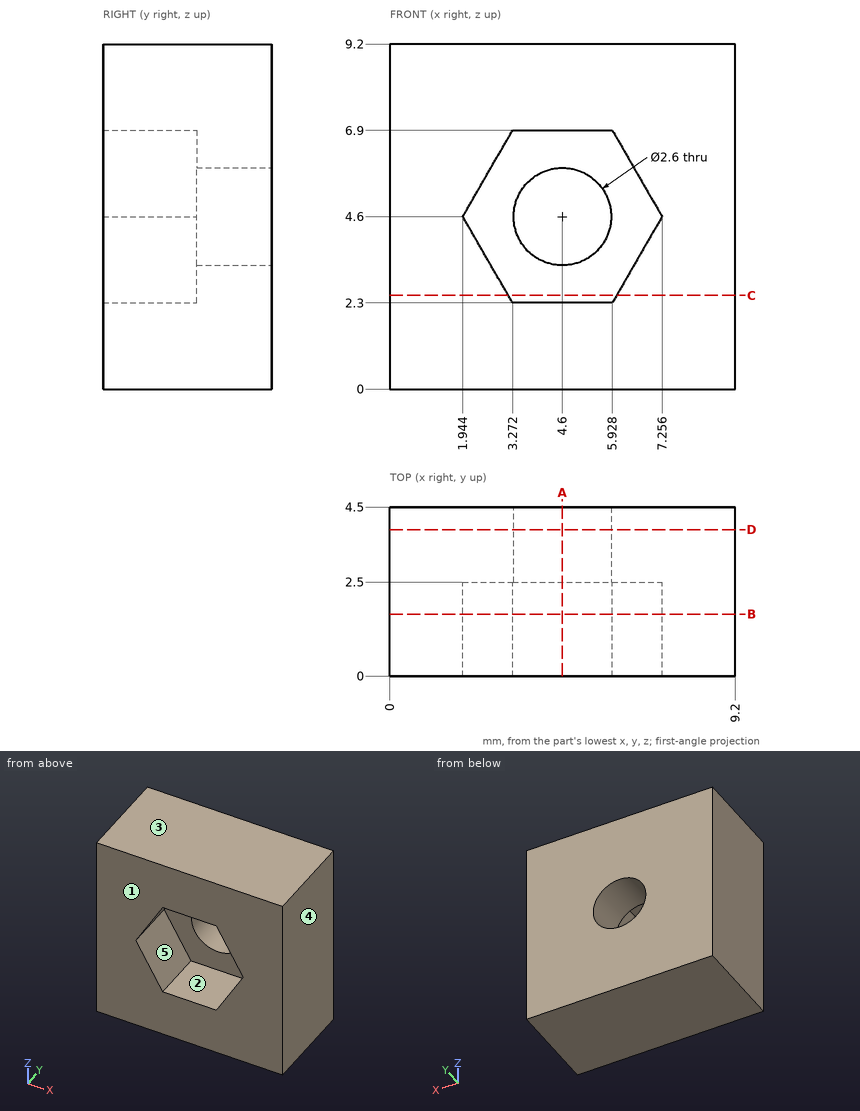
Study the drawing (mm; zero at the part's minimum x, y, z) and answer. A direction names the side the tool comes from. Give positions to 0.01 mm unless a question says otherwise; leave off trailing zeros. Order: outer loops, then holes, each group sorted by start corner. A loop starts at its lowest first (then second) coordinate and runs counter-clockwise, first axis right, second up.
1. Section B-B, the plane y = 1.65 is taken. Determine the outline of the cut face in (x, z).
Result sheet:
outline: (0, 0) - (9.2, 0) - (9.2, 9.2) - (0, 9.2) - close; hole (1.94, 4.6) - (3.27, 2.3) - (5.93, 2.3) - (7.26, 4.6) - (5.93, 6.9) - (3.27, 6.9) - close
2. The mould has two halves that part along X. Classify the marked faces 3, 4 and 5: released by +X, released by -X, zero draft, split by the parting line, or undercut.
Result sheet:
face 3: zero draft
face 4: released by +X
face 5: undercut
3. For the marked faces 1 and 2, determine the directions among +Z, -Z, +X, -X, +Y, -Y from which every point of the face is accessible in a straight line to the end or side of a thin tool.
Result sheet:
face 1: +Z, -Z, +X, -X, -Y
face 2: -Y
4. This flat-tipped pin is pushed along its axis until it touches: P1, Ø2, axis at x = 5, y = 1, coming from the -Z side. Where does it stop, or does it pass through?
Result sheet:
P1: stops at z = 0
5. Section A-A, the plane x = 4.6 is taken. Determine the outline of the cut face in (y, z), and give its area (3 significant figures).
Result sheet:
outline: (0, 0) - (4.5, 0) - (4.5, 3.3) - (2.5, 3.3) - (2.5, 2.3) - (0, 2.3) - close; (0, 6.9) - (2.5, 6.9) - (2.5, 5.9) - (4.5, 5.9) - (4.5, 9.2) - (0, 9.2) - close
area: 24.7 mm2
6. Section C-C, the plane z = 2.5 is taken. Determine the outline of the cut face in (x, y).
Result sheet:
outline: (0, 0) - (3.16, 0) - (3.16, 2.5) - (6.04, 2.5) - (6.04, 0) - (9.2, 0) - (9.2, 4.5) - (0, 4.5) - close
7. Straight lines are drawn through the part: L1, parallel to X at y = 3.7, z = 4.6; L2, parallel to Z at x = 4, y = 1.8. For each, find the intervals that lie inside material, in ascending order.
Result sheet:
L1: x = 0 to 3.3, 5.9 to 9.2
L2: z = 0 to 2.3, 6.9 to 9.2
8. Section D-D, the plane y = 3.9 is taken. Determine the outline of the cut face in (x, z), and give its area (3 significant figures).
Result sheet:
outline: (0, 0) - (9.2, 0) - (9.2, 9.2) - (0, 9.2) - close; hole circle Ø2.6 at (4.6, 4.6)
area: 79.3 mm2
